Autodesk Inventor part; units mm, degrees
ref_plane "YZ Plane" through (0, 0, 0) normal (1, 0, 0) x (0, 1, 0)
ref_plane "XZ Plane" through (0, 0, 0) normal (0, 1, 0) x (-1, 0, 0)
ref_plane "XY Plane" through (0, 0, 0) normal (0, 0, 1) x (1, 0, 0)
sketch "Sketch1" plane through (0, 0, 0) normal (0, 0, 1) x (1, 0, 0)
  line L0 (-1.39, -1.09) -> (1.39, -1.09)
  line L1 (1.39, -1.09) -> (1.39, -2.09)
  line L2 (1.39, -2.09) -> (-1.39, -2.09)
  line L3 (-1.39, -2.09) -> (-1.39, -1.09)
  point P0 (0, 0)
  dimension "d0" = 1
  dimension "d1" = 1.39
  dimension "d2" = 2.78
  dimension "d3" = 1.09
extrude "Extrusion1" add sketch "Sketch1" along normal blind 15.9
sketch "Sketch2" plane through (-1.39, -1.09, 0) normal (0, 1, 0) x (1, 0, 0)
  line L0 (0, 0) -> (0, -15.9)
  line L1 (0, -8.8) -> (2.78, -8.8)
  line L2 (2.78, -8.8) -> (2.78, -15.9)
  line L3 (2.78, -15.9) -> (0, -15.9)
  line L4 (0, -15.9) -> (0, -8.8)
  point P0 (1.39, 0)
  dimension "d6" = 7.1
extrude "Extrusion2" cut sketch "Sketch2" against normal blind 0.2685
sketch "Sketch3" plane through (0, 0, 0) normal (0, 0, -1) x (-1, 0, 0)
  line L0 (-1.39, -1.09) -> (1.39, -1.09)
  line L1 (1.39, -1.09) -> (1.39, 1.69)
  line L2 (1.39, 1.69) -> (-1.39, 1.69)
  line L3 (-1.39, 1.69) -> (-1.39, -1.09)
  point P0 (0, 0)
  dimension "d9" = 2.78
extrude "Extrusion3" add sketch "Sketch3" against normal blind 2
sketch "Sketch4" plane through (0, 0, 0) normal (0, 0, -1) x (-1, 0, 0)
  line L0 (-1.39, 1.69) -> (-1.39, -2.09)
  line L1 (1.39, -2.09) -> (1.39, 1.69)
  line L2 (1.39, 1.69) -> (-1.39, 1.69)
  circle A0 centre (0, 0) radius 0.8
  line L3 (-1.39, -1.3585) -> (1.39, -1.3585)
  line L4 (-1.39, -1.09) -> (1.39, -1.09)
  line L5 (-1.39, -1.09) -> (-0.7252, 0.3377)
  line L6 (1.39, -1.09) -> (0.7252, 0.3377)
  dimension "d12" = 1.6
extrude "Extrusion4" cut sketch "Sketch4" against normal through all contours L2 L1 L6 A0 L5 L0
sketch "Sketch5" plane through (0, 0, 0) normal (0, 0, -1) x (-1, 0, 0)
  line L0 (-0.7252, 0.3377) -> (-1.39, -1.09)
  line L1 (-1.39, -1.09) -> (-1.39, -2.09)
  line L2 (-1.39, -2.09) -> (1.39, -2.09)
  line L3 (1.39, -2.09) -> (1.39, -1.09)
  line L4 (1.39, -1.09) -> (0.7252, 0.3377)
  arc A0 (0.7252, 0.3377) -> (-0.7252, 0.3377) centre (0, 0) ccw
  circle A1 centre (0, 0) radius 0.8
extrude "Extrusion5" cut sketch "Sketch5" against normal blind 1 contours A1 L4 L3 L2 L1 L0
hole "Hole1" at (0, 0, 0) direction (0, 0, 1) diameter 0.4 end through all countersink diameter 0.8 countersink angle 90
sketch "Sketch6" plane through (-1.39, -2.09, 15.9) normal (0, -1, 0) x (1, 0, 0)
  line L0 (2.78, -15.9) -> (2.78, 0)
  line L1 (2.78, 0) -> (0, 0)
  circle A0 centre (1.39, -1.5) radius 0.5
  point P0 (2.78, -14.9)
  point P1 (1.39, -15.9)
  point P2 (1.39, -1)
  point P3 (1.39, -2)
  dimension "d26" = 1
  dimension "d27" = 1.39
  dimension "d28" = 1.5
extrude "Extrusion6" [suppressed]
chamfer "Chamfer1" distance 1 angle 45 1 edges at (0, -2.09, 1)
ref_plane "Work Plane1" through (0, -2.09, 14.9) normal (0, 0, 1) x (1, 0, 0)
ref_plane "Work Plane2" through (0, -2.09, 13.9) normal (0, 0, 1) x (1, 0, 0)
sketch "Sketch10" plane through (0, 0, 15.9) normal (0, 0, 1) x (1, 0, 0)
  line L0 (1.39, -1.3585) -> (-1.39, -1.3585)
  circle A0 centre (0, 0) radius 2.09
  line L1 (1.39, -2.09) -> (-1.39, -2.09)
  dimension "d54" = 4.18
extrude "Extrusion7" add sketch "Sketch10" against normal blind 0.9
sketch "Sketch11" plane through (0, 0, 15.9) normal (0, 0, 1) x (1, 0, 0)
  arc A0 (1.39, -1.5608) -> (-1.39, -1.5608) centre (0, 0) ccw
  circle A1 centre (0, 0) radius 1.3
  point P0 (1.6431, -0.954)
  point P1 (-1.6431, -0.954)
  dimension "d41" = 2.6
hole "Hole2" at (0, 0, 15.9) direction (0, 0, -1) diameter 3 depth 1.1
fillet "Fillet3" radius 0.7 2 edges at (1.39, -2.09, 8.95) (-1.39, -2.09, 8.95)
sketch "Sketch13" plane through (-1.39, -1.09, 8.8) normal (0, 0, 1) x (1, 0, 0)
  point P0 (1.39, 1.09)
  point P1 (1.39, 1.09)
hole "Hole4" at (0, 0, 8.8) at (0, 0, 8.8) direction (0, 0, -1) diameter 2.8 depth 6.8
sketch "Sketch15" plane through (0, -2.09, 14.9) normal (0, 0, 1) x (1, 0, 0)
  point P0 (0, 2.09)
  point P1 (0, 2.09)
hole "Hole5" [suppressed]
properties part number "MU_Motor_Asm_Frame_new3" material "Aluminum-6061"
Can you work these out from the model? Positions are in its coordinate system, mm. A direction names the side the tool comes from. Coordinates: 2 decimals unless noted, no trailing zeros. Write each loop counter-clockwise with the first axis right and the second up, starting at its lowest first coordinate (ties: lowest second). Pieces come first, ordered by that corner, then holes. Notation, with made-up numbers: (26, -37.75) - (32, -37.75) arc R23 ccw to (32, -1.75) - close; hole circle Ø10 at (-9, 43). An arc over 180 degrees is marked (long way). Return JSON: item names as keys, results as strings.
Q1. If we section it at A-A (x = 0): Please give me the cut outline in (y, z).
Computed values:
{"outline": "(-2.09, 2) - (-1.09, 1) - (-0.8, 1) - (-0.8, 0) - (-0.4, 0) - (-0.2, 0.2) - (-0.2, 2) - (-1.4, 2) - (-1.4, 8.8) - (-1.36, 8.8) - (-1.36, 14.8) - (-1.5, 14.8) - (-1.5, 15.9) - (-2.09, 15.9) - close; (0.2, 0.2) - (0.4, 0) - (0.8, 0) - (0.8, 2) - (0.2, 2) - close; (1.5, 15) - (2.09, 15) - (2.09, 15.9) - (1.5, 15.9) - close"}
Q2. Please list where these lines run through material, in increasing order: L1, parallel to X at y = 0, z = 15.35; L2, parallel to Y at x = 0, z = 0.95. Write a range as from..to.
Computed values:
{"L1": "x = -2.09..-1.5, 1.5..2.09", "L2": "y = -0.8..-0.2, 0.2..0.8"}
Q3. If we section it at C-C (z = 7.75): Please give me the cut outline in (x, y), then the cut area to 3 significant figures.
Computed values:
{"outline": "(-1.39, -1.39) arc R0.7 ccw to (-0.69, -2.09) - (0.69, -2.09) arc R0.7 ccw to (1.39, -1.39) - (1.39, -1.09) - (0.88, -1.09) arc R1.4 cw to (-0.88, -1.09) - (-1.39, -1.09) - close", "area": "2.20 mm2"}
Q4. If we section it at D-D (x = -1.2): Please give me the cut outline in (y, z), then the cut area to 3 significant figures.
Computed values:
{"outline": "(-1.87, 1.78) - (-1.09, 1) - (-0.68, 1) - (-0.68, 2) - (-1.09, 2) - (-1.09, 8.8) - (-1.36, 8.8) - (-1.36, 15) - (-0.9, 15) - (-0.9, 15.9) - (-1.87, 15.9) - close; (0.9, 15) - (1.71, 15) - (1.71, 15.9) - (0.9, 15.9) - close", "area": "11.0 mm2"}
Q5. If we section it at B-B (y = 0): Please give me the cut outline in (x, z), then the cut area to 3 significant figures.
Computed values:
{"outline": "(-2.09, 15) - (-1.5, 15) - (-1.5, 15.9) - (-2.09, 15.9) - close; (-0.88, 1) - (-0.8, 1) - (-0.8, 0) - (-0.4, 0) - (-0.2, 0.2) - (-0.2, 2) - (-0.88, 2) - close; (0.2, 0.2) - (0.4, 0) - (0.8, 0) - (0.8, 1) - (0.88, 1) - (0.88, 2) - (0.2, 2) - close; (1.5, 15) - (2.09, 15) - (2.09, 15.9) - (1.5, 15.9) - close", "area": "3.59 mm2"}
Q6. Thinking about a two-plate mould opening in X: for faces 5 (the cylindrical face through (0.575, -1.386, 15.465)), 6 (the flat face through (1.062, -0.386, 1.493)), 7 (the cylindrical face through (0, -1.4, 5.4)), 8 (the flat face through (-0.9, 1.5, 15)), which applies, +X half, -X half, draft (parallel to the pull), parting line (faces both ways), or undercut?
Computed values:
{"face 5": "undercut", "face 6": "+X half", "face 7": "undercut", "face 8": "draft"}
Q7. I'm going to push flat-ended pins straight in: pin 1 Ø1 at (x, z) = (1.5, 14) entering from -Y; pin 2 Ø1 at (x, z) = (-1, 4.5) entering from +Y; pin 3 Ø1 at (y, z) = (-1, 14) entering from +X. Where does each tip first touch, or does it pass through?
Computed values:
{"pin 1": "stops at y = -2.02", "pin 2": "stops at y = -1.09", "pin 3": "stops at x = 1.39"}
Q8. On a 3-axis mill with a long thin cutter (end or side, diameter ignored), from which of +Z, -Z, +X, -X, +Y, -Y can I reach the whole of each face in a straight line? I mean faces 1 (the flat face through (0, -1.358, 12)), 2 (the flat face through (-1.062, -0.386, 1.493)), 3 (the cylindrical face through (0.104, 0.793, 0.764)), 4 (the flat face through (0, -2.09, 9)). Say none if no direction works.
Computed values:
{"face 1": "+X, -X, +Y", "face 2": "-Z, -X, +Y", "face 3": "-Z", "face 4": "+Z, -Z, +X, -X, -Y"}
